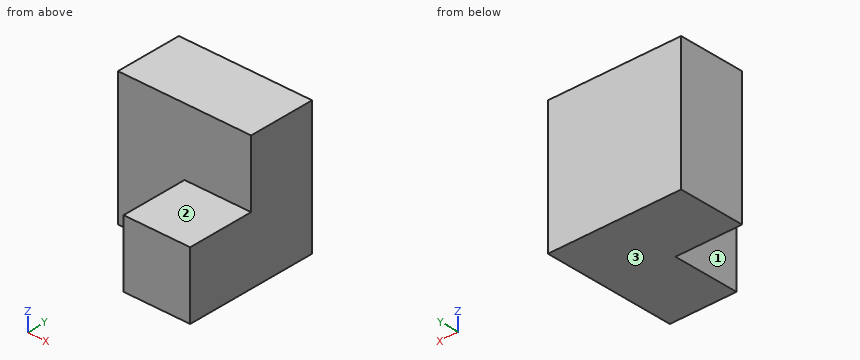
from build123d import *

# Parameters (mm, degrees)
F1_W     = 25.4
F1_H     = 25.4
F2_DEPTH = 50.8
F0_W     = 50.8
F0_H     = 50.8
F3_DEPTH = 25.4
F4_DEPTH = 25.4


with BuildPart() as f2:
    # F1 (on face) → F2 (new body)
    with BuildSketch(Plane.XZ):
        with Locations((-12.7, 12.7)):
            Rectangle(F1_W, F1_H)
    extrude(amount=F2_DEPTH)

    # F0 (on Front) → F3 (join)
    with BuildSketch(Plane.XZ):
        with Locations((-25.4, 25.4)):
            Rectangle(F0_W, F0_H)
    extrude(amount=F3_DEPTH)

    # F0 (on Front) → F4 (join)
    with BuildSketch(Plane.XZ):
        with Locations((-25.4, 25.4)):
            Rectangle(F0_W, F0_H)
    extrude(amount=F4_DEPTH)


solid = f2.part
The listing builds one solid part. Answer for the finished solid, in the listing's coordinates (mm). Face numbers are marked on the shaded views. A direction names the side the tool comes from. Round coordinates to 2 decimals unless told otherwise and drop trailing zeros. Write each loop counter-clockwise with the first axis right and the second up, starting at its lowest first coordinate (ties: lowest second). Pieces come first, ordered by that corner, then holes. Notation, with made-up numbers: (22.5, 47.5) - (75.5, 47.5) arc R10 cw to (75.5, 55.5) - close; hole circle Ø4 at (2.25, -5). An arc over 180 degrees is marked (long way). Use a Markdown table: item, result. Add a question column.
1. A tool of negligible diameter and unlimited length cuts with its end or side. For the marked faces 1, 2 and 3, from which of +Z, -Z, +X, -X, +Y, -Y can it reach the whole face along a straight path? Write none if from no direction.
2. The part is cut by section D-D (z = 30.5). Write down the section's boundary in (x, y).
3. Consider line 1 (Y direction, x = -33, z = 46.5); line 2 (Z direction, x = -20, y = -46). Determine where each line is inside the solid, lowest interval first.
4. The part is cut by section A-A (z = 16). Write down the section's boundary in (x, y), and give its area (3 significant figures).
5. The part is cut by section B-B (x = -11.5). Write down the section's boundary in (y, z).
6. Flat-ended cylindrical pins translate along their axes: P1, Ø5, axis at x = -6.5, z = 35.5, coming from the -Y side; P2, Ø1, axis at y = -34.5, z = 18, coming from the -X side; P3, Ø20.5, axis at x = -8, y = -38, coming from the +Z side. Find the tip coordinate at first contact, or state that the pin passes through.
7. The part is cut by section C-C (y = -35). Write down the section's boundary in (x, z).
Reported:
| question | item | result |
|---|---|---|
| 1 | face 1 | +Z, -Z, -X, -Y |
| 1 | face 2 | +Z, +X, -X, -Y |
| 1 | face 3 | -Z, +X, -X, +Y, -Y |
| 2 | outline | (-50.8, -25.4) - (0, -25.4) - (0, 0) - (-50.8, 0) - close |
| 3 | line 1 | -25.4 to 0 |
| 3 | line 2 | 0 to 25.4 |
| 4 | outline | (-50.8, -25.4) - (-25.4, -25.4) - (-25.4, -50.8) - (0, -50.8) - (0, 0) - (-50.8, 0) - close |
| 4 | area | 1,940 mm^2 |
| 5 | outline | (-50.8, 0) - (0, 0) - (0, 50.8) - (-25.4, 50.8) - (-25.4, 25.4) - (-50.8, 25.4) - close |
| 6 | P1 | y = -25.4 |
| 6 | P2 | x = -25.4 |
| 6 | P3 | z = 25.4 |
| 7 | outline | (-25.4, 0) - (0, 0) - (0, 25.4) - (-25.4, 25.4) - close |
